Geometry check sheet. Reference: the model listing, model coordinates, mm. A direction names the side the tool comes from. Round coordinates to 2 decimals unless told otherwise and drop trailing zeros. Write each loop counter-clockwise with the first axis right and the second up, starting at its lowest first coordinate (ties: lowest second). Pieces come first, ordered by that corner, then holes. Notation, with made-up numbers: M 27.25,52.5 L 82.25,52.5 A29 ccw 82.25,75.5 Z; hole C -28,62.5 d5. An arc over 180 degrees is marked long. Put each result on its own line as item: value. Start each with the question number.
(1) Section check A-A on y = 1.15. Record the cut outline in (x, z).
(2) Material ranges on probe 1 along Z at (x, y) = (18.5, 0.95); probe 2 along X at (y, z) = (2.3, -21); probe 3 along Z at (x, y) = (-16, 0.8), recorded low to high.
(3) Section check C-C on z = -21. Record the cut outline in (x, y), then the cut area to 3 significant figures.
(4) Section check B-B on x = 18.5. Record the cut outline in (y, z), then the cut area to 3 significant figures.
(5) Mould release check, pull along X, two halves, no side actions. Record for faces 1 (the flat face through (32, 1, 6)), 2 (the flat face through (-16, 2, -32)), 3 (the flat face through (8, 1, 8)), 4 (the flat face through (-24, 1, 8)): pulls with the +X half, pulls with the -X half, needs draft (parallel to the pull), parting line crosses it, or undercut.
(6) Gauge pin test, flat ends, axial feed: pin 1 (1.5 mm diameter, centred on x = 0, y = 1.5, fed in from +Z); pin 2 (1.5 mm diameter, centred on y = 1, z = 7.5, fed in from -X); pin 3 (4 mm diameter, centred on x = 18.5, z = -21, fed in from -Y); pin 4 (1.5 mm diameter, centred on y = 2, z = -40, fed in from -X). Record the tip position at first contact, or that the pin passes through.
(7) Tool access check on faces 5 (the flat face through (8, 2, -33)), 6 (the flat face through (24, 1, 7)), 7 (the flat face through (-37, 1, -42)). Record the directions out of +Z, -Z, +X, -X, +Y, -Y that give a thin tool (end or side, any length) a straight path to the whole face; none if there is none.
(8) Section check D-D on z = -41. Record the cut outline in (x, y).
from build123d import *

# Parameters (mm, degrees)
BOSS_EXTRUDE1_DEPTH = 3
SKETCH2_R           = 1.6
SKETCH2_W           = 4
SKETCH2_H           = 3
SKETCH2_W_2         = 16
CUT_EXTRUDE1_DEPTH  = 4


with BuildPart() as part:
    # Sketch1 → Boss-Extrude1 (new body)
    with BuildSketch(Plane(origin=(0, 0, 0), x_dir=(1, 0, 0), z_dir=(0, 1, 0))):
        Polygon((-40, 37), (-34, 47), (34, 47), (40, 37), (40, -6), (24, -6), (24, -9), (8, -9), (8, -6), (-8, -6), (-8, -9), (-24, -9), (-24, -6), (-40, -6), align=None)
    extrude(amount=BOSS_EXTRUDE1_DEPTH)

    # Sketch2 → Cut-Extrude1 (cut, through all)
    with BuildSketch(Plane(origin=(0, 3, 0), x_dir=(1, 0, 0), z_dir=(0, 1, 0))):
        with Locations((-18.5, 21)):
            Circle(SKETCH2_R)
        with Locations((18.5, 21)):
            Circle(SKETCH2_R)
        with Locations((0, 3)):
            Rectangle(SKETCH2_W, SKETCH2_H)
        with Locations((-16, 33.5)):
            Rectangle(SKETCH2_W_2, SKETCH2_H)
        with Locations((16, 33.5)):
            Rectangle(SKETCH2_W_2, SKETCH2_H)
    extrude(amount=-CUT_EXTRUDE1_DEPTH, mode=Mode.SUBTRACT)


solid = part.part
Answers follow:
1. outline: M -40,-37 L -34,-47 L 34,-47 L 40,-37 L 40,6 L 24,6 L 24,9 L 8,9 L 8,6 L -8,6 L -8,9 L -24,9 L -24,6 L -40,6 Z; hole M -24,-35 L -8,-35 L -8,-32 L -24,-32 Z; hole C -18.5,-21 d3.2; hole M -2,-4.5 L 2,-4.5 L 2,-1.5 L -2,-1.5 Z; hole M 8,-35 L 24,-35 L 24,-32 L 8,-32 Z; hole C 18.5,-21 d3.2
2. probe 1: z = -47 to -35, -32 to -22.6, -19.4 to 9
2. probe 2: x = -40 to -20.1, -16.9 to 16.9, 20.1 to 40
2. probe 3: z = -47 to -35, -32 to 9
3. outline: M -40,0 L -20.1,0 L -20.1,3 L -40,3 Z; M -16.9,0 L 16.9,0 L 16.9,3 L -16.9,3 Z; M 20.1,0 L 40,0 L 40,3 L 20.1,3 Z
3. area: 221 mm^2
4. outline: M 0,-47 L 3,-47 L 3,-35 L 0,-35 Z; M 0,-32 L 3,-32 L 3,-22.6 L 0,-22.6 Z; M 0,-19.4 L 3,-19.4 L 3,9 L 0,9 Z
4. area: 149 mm^2
5. face 1: needs draft
5. face 2: undercut
5. face 3: undercut
5. face 4: pulls with the -X half
6. pin 1: stops at z = 6
6. pin 2: stops at x = -24
6. pin 3: stops at y = 0
6. pin 4: stops at x = -38.65
7. face 5: +Y, -Y
7. face 6: +Z, +X, +Y, -Y
7. face 7: -Z, -X, +Y, -Y
8. outline: M -37.6,0 L 37.6,0 L 37.6,3 L -37.6,3 Z
